Print and shaded views of the part. All mm, measured from the part's lowest x, y and z. Coordinates: 2 decimals unless noted, no trailing zeros. Loops run counter-clockwise (first coordinate to the right, second up) from the corner with the lowest first, then second, coordinate; pieces in that order, holes last.
1) Saw through at A-A, the plane z = 3.75. Write the cut outline in (x, y).
2) Saw through at D-D, the plane x = 22.5. Write the cut outline in (y, z), and give its area (3 significant figures).
3) Saw through at B-B, the plane x = 54.5. Write the cut outline in (y, z), and give its area (3 significant figures).
4) Two-plate mould, pull along X, no slides. Class the marked faces 1, 2 and 3: +X half, -X half, draft (parallel to the pull), parting line (faces both ways), or undercut.
5) Pin check, flat tips, straight feed: pin 1 Ø3 at (y, z) = (5.5, 6) entering from +X; pin 2 Ø4 at (x, y) = (13.5, 4) entering from -Z; pin 3 Ø2 at (y, z) = (3, 1) entering from +X. Stop position of each tip, or through.
6) Saw through at C-C, the plane z = 8.25. Write the cut outline in (x, y), and give its area (3 significant figures).
7) Wall check: line 1 along Y through (x, z) = (6, 8.2); line 2 along X through (y, z) = (7.5, 9.25); line 3 along X through (y, z) = (6.75, 6.5). Give the ranges that are in metal, low to high.
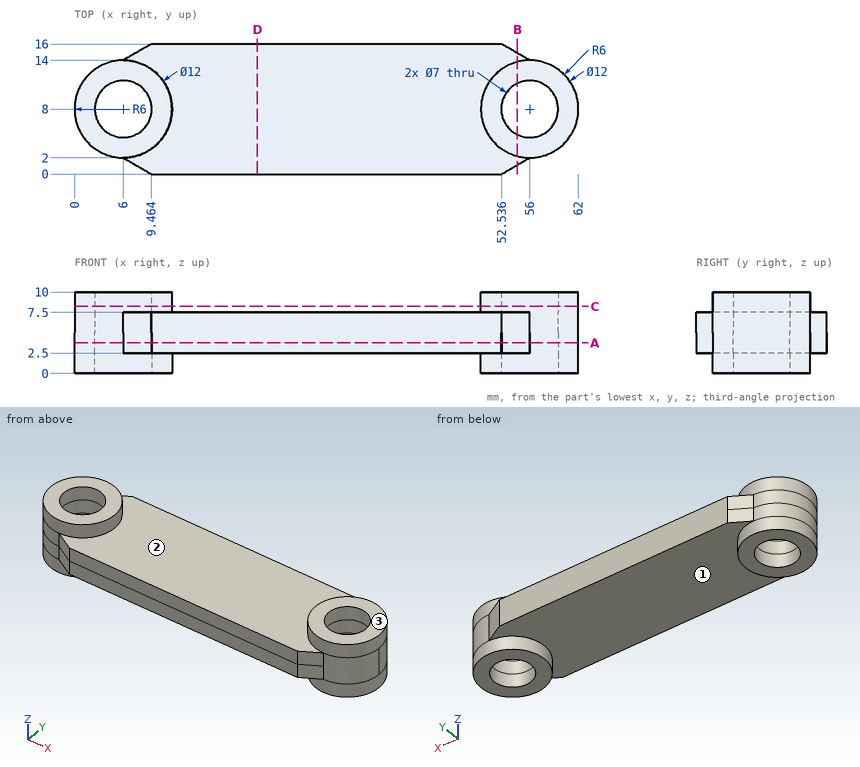
Data:
1. outline: (6, 2) - (9.46, 0) - (52.54, 0) - (56, 2) arc R6 ccw to (56, 14) - (52.54, 16) - (9.46, 16) - (6, 14) arc R6 ccw to start; hole circle Ø7 at (6, 8); hole circle Ø7 at (56, 8)
2. outline: (0, 2.5) - (16, 2.5) - (16, 7.5) - (0, 7.5) - close
2. area: 80.0 mm2
3. outline: (1.13, 2.5) - (2.19, 2.5) - (2.19, 0) - (4.84, 0) - (4.84, 10) - (2.19, 10) - (2.19, 7.5) - (1.13, 7.5) - close; (11.16, 0) - (13.81, 0) - (13.81, 2.5) - (14.87, 2.5) - (14.87, 7.5) - (13.81, 7.5) - (13.81, 10) - (11.16, 10) - close
3. area: 63.5 mm2
4. face 1: undercut
4. face 2: undercut
4. face 3: draft
5. pin 1: stops at x = 61.92
5. pin 2: stops at z = 2.5
5. pin 3: stops at x = 60.47
6. outline: circle Ø12 at (6, 8); circle Ø12 at (56, 8); hole circle Ø7 at (6, 8); hole circle Ø7 at (56, 8)
6. area: 149 mm2
7. line 1: y = 2 to 4.5, 11.5 to 14
7. line 2: x = 0.02 to 2.54, 9.46 to 11.98, 50.02 to 52.54, 59.46 to 61.98
7. line 3: x = 0.13 to 2.73, 9.27 to 52.73, 59.27 to 61.87
